Can you work these out from the model? Positions are in its coordinate system, mm. Face numbers are marked on the shaded views. Round coordinates to 2 decimals unless told otherwise and drop trailing zeros. Order: outer loops, then holes, each group sorted by start corner. A loop starts at its lowest first (then second) coordinate and runs counter-clockwise, first axis right, second up.
Q1. If I drill on line 1 (Z direction, x = 3.8, y = 0); line 2 (X direction, y = 8.5, z = 14); line 3 (Z direction, x = 4.35, y = 5), over which ranges is the centre line in solid material (lowest first)?
Q2. If we section it at C-C (x = 4.05): Please give me the cut outline in (y, z), plus the area to 3 significant figures.
Q3. If we section it at A-A (z = 0): Please give me the cut outline in (x, y), plus the area to 3 significant figures.
Q4. We'd pull the mould along Z, two halves only. Please class the marked faces 1, 2, 3 and 4: pulls with the +Z half, pulls with the -Z half, needs draft (parallel to the pull), parting line crosses it, or undercut.
Q5. If we section it at B-B (y = 0): Please give me the cut outline in (x, z).
Q6. Will these pins go through, and if not, where does the flat tip stop? P1, Ø3, axis at x = 2, y = -8.5, coming from the +Z side; P2, Ø1.5, axis at x = 3, y = -10, coming from the -Z side.
Q7. If we section it at D-D (z = 12.5): Please give me the cut outline in (x, y).
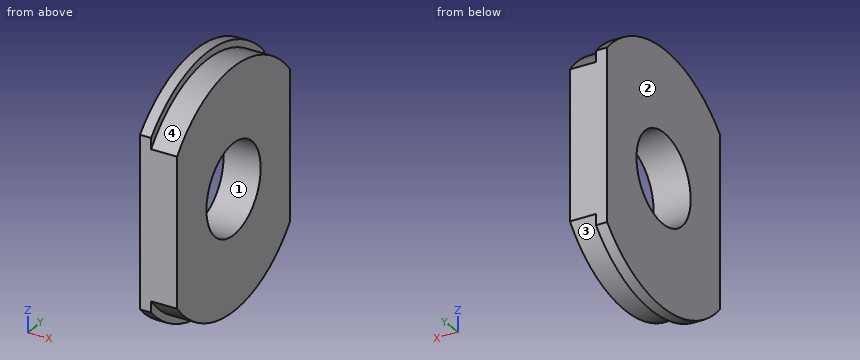
from build123d import *

# Parameters (mm, degrees)
F3_D     = 12
F5_DEPTH = 25


with BuildPart() as f1:
    # F0 (on Front) → F1 (revolve)
    with BuildSketch(Plane.XZ):
        Polygon((0, 16.9), (0, 0), (5, 0), (5, 15.95), (1.5, 15.95), (1.5, 16.9), align=None)
    revolve(axis=Axis((2.5, 0, 0), (1, 0, 0)))

    # F3 (through all)
    with Locations(Plane.YZ.offset(5)):
        with Locations((0, 0)):
            Hole(F3_D / 2)

    # F4 (on face) → F5 (cut)
    with BuildSketch(Plane.YZ.offset(5)):
        with BuildLine():
            Line((-12.5, -9.9071943556), (-12.5, 9.9071943556))
            ThreePointArc((-12.5, 9.9071943556), (-15.95, 0), (-12.5, -9.9071943556))
        make_face()
        with BuildLine():
            Line((-12.5, 9.9071943556), (-12.5, 11.3736537665))
            ThreePointArc((-12.5, 11.3736537665), (-16.9, 0), (-12.5, -11.3736537665))
            Line((-12.5, -11.3736537665), (-12.5, -9.9071943556))
            ThreePointArc((-12.5, -9.9071943556), (-15.95, 0), (-12.5, 9.9071943556))
        make_face()
        with BuildLine():
            ThreePointArc((15.95, 0), (15.0628267599, 5.2453550881), (12.5, 9.9071943556))
            Line((12.5, 9.9071943556), (12.5, -9.9071943556))
            ThreePointArc((12.5, -9.9071943556), (15.0628267599, -5.2453550881), (15.95, 0))
        make_face()
        with BuildLine():
            ThreePointArc((12.5, -11.3736537665), (15.7616623489, -6.0975404878), (16.9, 0))
            ThreePointArc((16.9, 0), (15.7616623489, 6.0975404878), (12.5, 11.3736537665))
            Line((12.5, 11.3736537665), (12.5, 9.9071943556))
            ThreePointArc((12.5, 9.9071943556), (15.0628267599, 5.2453550881), (15.95, 0))
            ThreePointArc((15.95, 0), (15.0628267599, -5.2453550881), (12.5, -9.9071943556))
            Line((12.5, -9.9071943556), (12.5, -11.3736537665))
        make_face()
    extrude(amount=-F5_DEPTH, mode=Mode.SUBTRACT)


solid = f1.part
Solution:
1. line 1: z = -15.95 to -6, 6 to 15.95
1. line 2: x = 0 to 1.5
1. line 3: z = -15.15 to -3.32, 3.32 to 15.15
2. outline: (-12.5, -9.91) arc R15.95 ccw to (12.5, -9.91) - (12.5, 9.91) arc R15.95 ccw to (-12.5, 9.91) - close; hole circle Ø12 at (0, 0)
2. area: 593 mm2
3. outline: (0, -12.5) - (5, -12.5) - (5, -6) - (0, -6) - close; (0, 6) - (5, 6) - (5, 12.5) - (0, 12.5) - close
3. area: 65.0 mm2
4. face 1: undercut
4. face 2: needs draft
4. face 3: pulls with the -Z half
4. face 4: pulls with the +Z half
5. outline: (0, -16.9) - (1.5, -16.9) - (1.5, -15.95) - (5, -15.95) - (5, -6) - (0, -6) - close; (0, 6) - (5, 6) - (5, 15.95) - (1.5, 15.95) - (1.5, 16.9) - (0, 16.9) - close
6. P1: stops at z = 15.34
6. P2: stops at z = -12.99
7. outline: (0, -11.37) - (1.5, -11.37) - (1.5, -9.91) - (5, -9.91) - (5, 9.91) - (1.5, 9.91) - (1.5, 11.37) - (0, 11.37) - close
